Autodesk Inventor part; units mm, degrees
ref_plane "YZ Plane" through (0, 0, 0) normal (1, 0, 0) x (0, 1, 0)
ref_plane "XZ Plane" through (0, 0, 0) normal (0, 1, 0) x (-1, 0, 0)
ref_plane "XY Plane" through (0, 0, 0) normal (0, 0, 1) x (1, 0, 0)
sketch "Skizze1" plane through (0, 0, 0) normal (0, 0, 1) x (1, 0, 0)
  line L0 (-4.9, 0) -> (4.9, 0)
  line L1 (0, -44.8) -> (0, 44.8)
  line L2 (0, 5) -> (0, -5) construction
  line L3 (2.5, 5) -> (2.5, -5)
  line L4 (-2.5, -5) -> (-2.5, 5)
  arc A0 (2.5, 5) -> (-2.5, 5) centre (0, 5) ccw
  arc A1 (-2.5, -5) -> (2.5, -5) centre (0, -5) ccw
  line L5 (0, 28.5) -> (0, -28.5) construction
  line L6 (-3.5, 28.5) -> (-3.5, -28.5)
  line L7 (3.5, -28.5) -> (3.5, 28.5)
  arc A2 (3.5, 28.5) -> (-3.5, 28.5) centre (0, 28.5) ccw
  arc A3 (-3.5, -28.5) -> (3.5, -28.5) centre (0, -28.5) ccw
  line L8 (0, 12.5) -> (0, 22.5) construction
  line L9 (2.5, 12.5) -> (2.5, 22.5)
  line L10 (-2.5, 22.5) -> (-2.5, 12.5)
  arc A4 (-2.5, 12.5) -> (2.5, 12.5) centre (0, 12.5) ccw
  arc A5 (2.5, 22.5) -> (-2.5, 22.5) centre (0, 22.5) ccw
  line L11 (0, -22.5) -> (0, -12.5) construction
  line L12 (2.5, -22.5) -> (2.5, -12.5)
  line L13 (-2.5, -12.5) -> (-2.5, -22.5)
  arc A6 (-2.5, -22.5) -> (2.5, -22.5) centre (0, -22.5) ccw
  arc A7 (2.5, -12.5) -> (-2.5, -12.5) centre (0, -12.5) ccw
  point P0 (0, 0)
  point P1 (0, 0)
  point P2 (0, 0)
  point P3 (0, 17.5)
  point P4 (0, -17.5)
  dimension "d0" = 5
  dimension "d1" = 15
  dimension "d2" = 7
  dimension "d3" = 10
  dimension "d4" = 10
  dimension "d5" = 32
  dimension "d31" = 2.5
extrude "Extrusion1" add sketch "Skizze1" along normal blind 0.5 contours L6 A2 L1 A5 L10 A4 A0 L4 L0 | L0 L4 A1 L1 A7 L13 A6 A3 L6 | A2 L7 L0 L3 A0 L1 A4 L9 A5 | L1 A6 L12 A7 A1 L3 L0 L7 A3
sketch "Skizze2" plane through (0, 0, 0) normal (0, 0, -1) x (-1, 0, 0)
  line L0 (3.5, 28.5) -> (3.5, -28.5)
  arc A0 (3.5, 28.5) -> (-3.5, 28.5) centre (0, 28.5) ccw
  line L1 (-3.5, -28.5) -> (-3.5, 28.5)
  arc A1 (-3.5, -28.5) -> (3.5, -28.5) centre (0, -28.5) ccw
  point P0 (0, 0)
extrude "Extrusion2" add sketch "Skizze2" along normal blind 1
sketch "Skizze3" plane through (0, 0, 0.5) normal (0, 0, 1) x (1, 0, 0)
  arc A0 (-3.5, -28.5) -> (3.5, -28.5) centre (0, -28.5) ccw
  arc A1 (3.5, 28.5) -> (-3.5, 28.5) centre (0, 28.5) ccw
  point P0 (0, 0)
hole "Bohrung1" at (0, 28.5, 0.5) at (0, -28.5, 0.5) direction (0, 0, -1) diameter 2.4 end through all countersink diameter 4.6 countersink angle 90
sketch "Skizze5" plane through (0, 0, 0) normal (0, 0, 1) x (1, 0, 0)
  arc A0 (-2.5, -22.5) -> (2.5, -22.5) centre (0, -22.5) ccw
  line L0 (2.5, -22.5) -> (2.5, -12.5)
  arc A1 (2.5, -12.5) -> (-2.5, -12.5) centre (0, -12.5) ccw
  line L1 (0, -15.5) -> (0, -19.5) construction
  line L2 (2, -15.5) -> (2, -19.5)
  line L3 (-2, -19.5) -> (-2, -15.5)
  arc A2 (2, -15.5) -> (-2, -15.5) centre (0, -15.5) ccw
  arc A3 (-2, -19.5) -> (2, -19.5) centre (0, -19.5) ccw
  line L4 (0, -22.5) -> (0, -12.5)
  line L5 (0, -12.5) -> (0, -17.5)
  line L6 (-1.3218, -17.5) -> (0, -17.5)
  point P0 (0, 0)
  point P1 (0, -17.5)
  dimension "d24" = 4
  dimension "d25" = 8
extrude "Extrusion3" cut sketch "Skizze5" against normal through all
pattern_linear "Rechteckige Anordnung1" count 3 spacing 17.5 along (0, 1, 0) of "Extrusion3"
properties part number "13_1087_018"
For this review, take the finished solid that the model builds, in its own axes (mm). A direction names the side the tool comes from. Coordinates: 2 decimals unless noted, no trailing zeros. Loops run counter-clockwise (first coordinate to the right, second up) from the corner with the lowest first, then second, coordinate; pieces in that order, holes last. Notation, with made-up numbers: (63, 28) - (114, 28) arc R28 ccw to (114, 47) - close; hole circle Ø10 at (-35, -6). An arc over 180 degrees is marked (long way). Return JSON: item names as keys, results as strings.
Item 1: Take a section at B-B (y = -24). Give the boundary of the cut face in (x, z).
Determined:
{"outline": "(-3.5, -1) - (3.5, -1) - (3.5, 0.5) - (2, 0.5) - (2, 0) - (-2, 0) - (-2, 0.5) - (-3.5, 0.5) - close"}
Item 2: Insertion check: pin 1 (2.5 mm diameter, centred on x = 0, y = 3, fed in from +Z); pin 2 (2 mm diameter, centred on x = 0, y = -28.5, fed in from -Z). Each pin has a flat end and moves straight along its axis. Give the tip position at first contact, or say it passes through.
Determined:
{"pin 1": "stops at z = 0", "pin 2": "passes through"}
Item 3: For faces 1 (the cylindrical face through (0, -4, -0.5)), 2 (the flat face through (-3.5, 0, 0)), 3 (the cylindrical face through (-0.1, 7.5, 0.2)), list the 3-axis set-ups (+Z, -Z, +X, -X, +Y, -Y) from which the entire face can be reached by the end or side of a thin tool; tool diameter is ignored.
Determined:
{"face 1": "+Z, -Z", "face 2": "+Z, -Z, -X, +Y, -Y", "face 3": "+Z"}
Item 4: Mouldability with a two-part tool opening along Y and no side actions: class faces 4 (the cylindrical face through (0.1, -7.5, 0.2)), 5 (the flat face through (-2.3, 0.4, -1)), 6 (the cylindrical face through (0, 32, 0)) as pulls with the +Y half, pulls with the -Y half, needs draft (parallel to the pull), parting line crosses it, or undercut.
Determined:
{"face 4": "undercut", "face 5": "needs draft", "face 6": "pulls with the +Y half"}
Item 5: For line 1 (Y direction, x = 0, z = -0.85); line 2 (X direction, y = 28.5, z = -0.7); line 3 (Y direction, x = -1.5, z = 0.2), list the stretches that pass through material, from the lowest coordinate up.
Determined:
{"line 1": "y = -32 to -29.7, -27.3 to -21.5, -13.5 to -4, 4 to 13.5, 21.5 to 27.3, 29.7 to 32", "line 2": "x = -3.5 to -1.2, 1.2 to 3.5", "line 3": "y = -31.66 to -29.82, -27.18 to -24.5, -10.5 to -7, 7 to 10.5, 24.5 to 27.18, 29.82 to 31.66"}
Item 6: Take a section at A-A (y = -0.5). Give the boundary of the cut face in (x, z).
Determined:
{"outline": "(-3.5, -1) - (-2, -1) - (-2, 0) - (-2.5, 0) - (-2.5, 0.5) - (-3.5, 0.5) - close; (2, -1) - (3.5, -1) - (3.5, 0.5) - (2.5, 0.5) - (2.5, 0) - (2, 0) - close"}
